Read the model definition and answer for the solid it produces. Units are mm, in the model's axes. A direction names the side the tool comes from. Give positions to 0.01 mm unless a question says otherwise; leave off trailing zeros. Order: outer loops, then holes, each group sorted by start corner. A loop starts at its lowest first (then second) coordinate and runs counter-clockwise, first axis right, second up. Notation, with made-up numbers: (64.5, 42.5) - (70.5, 42.5) arc R22 ccw to (70.5, 69.5) - close; hole circle Ø7 at (-3, 84.5). An arc over 180 degrees is marked (long way). Return JSON: item names as keys, results as strings.
```python
from build123d import *

# Parameters (mm, degrees)
SKETCH_1_R           = 10
EXTRUDE_1_DEPTH      = 250
SKETCH_3_W           = 1.3
SKETCH_3_H           = 0.5
SKETCH_4_OUTSIDE_W   = 122.16
SKETCH_4_OUTSIDE_H   = 122.16
SKETCH_4_OUTSIDE_W_2 = 15
SKETCH_4_OUTSIDE_H_2 = 51.001115416
CUT_EXTRUDE_1_DEPTH  = 10


with BuildPart() as part:
    # 草图1 → 凸台-拉伸1 (new, symmetric)
    with BuildSketch(Plane.XY):
        Circle(SKETCH_1_R)
    extrude(amount=EXTRUDE_1_DEPTH, both=True)

    # 草图3 → 切除-旋转1 (revolve, cut)
    with BuildSketch(Plane(origin=(100, 0, 250), x_dir=(0, 0, -1), z_dir=(0, 1, 0))):
        with Locations((24.45, 90.25)):
            Rectangle(SKETCH_3_W, SKETCH_3_H)
    cut_revolve_1 = revolve(axis=Axis((0, 0, 250), (0, 0, -1)), mode=Mode.SUBTRACT)

    # 草图4 outside → 切除-拉伸1 (cut)
    with BuildSketch(Plane(origin=(0, 0, -250), x_dir=(-1, 0, 0), z_dir=(0, 0, -1))):
        Rectangle(SKETCH_4_OUTSIDE_W, SKETCH_4_OUTSIDE_H)
        Rectangle(SKETCH_4_OUTSIDE_W_2, SKETCH_4_OUTSIDE_H_2, mode=Mode.SUBTRACT)
    cut_extrude_1 = extrude(amount=-CUT_EXTRUDE_1_DEPTH, mode=Mode.SUBTRACT)

    # 镜向1: 切除-旋转1, 切除-拉伸1 across plane
    add(cut_revolve_1.mirror(Plane.XY), mode=Mode.SUBTRACT)
    add(cut_extrude_1.mirror(Plane.XY), mode=Mode.SUBTRACT)


solid = part.part
```
Q1. Consider L1, parallel to X at y = 0.75, z = -29.5; L2, parallel to Y at x = 6.5, z = 188; L3, parallel to Y at x = -7.5, z = 171.5. Determine where each line is inside the solid, lowest interval first.
Values:
{"L1": "x = -9.97 to 9.97", "L2": "y = -7.6 to 7.6", "L3": "y = -6.61 to 6.61"}
Q2. Determine the mould class of faces 6 (the flat face through (9, 4, -226.2)), 7 (the cylindrical face through (-1.302, 9.915, -235.289)), 8 (the flat face through (0, 0, -250)) for opening direction Z: released by +Z, released by -Z, zero draft, split by the parting line, or undercut.
Values:
{"face 6": "undercut", "face 7": "zero draft", "face 8": "released by -Z"}
Q3. A cutting plane is placed at A-A (z = -213). Write down the section's boundary in (x, y).
Values:
{"outline": "circle Ø20 at (0, 0)"}
Q4. Given pin 1 (5 mm diameter, centred on y = 0.5, z = -245.5, fed in from -X); pin 2 (1.2 mm diameter, centred on x = -8.5, y = 0, fed in from -Z); pin 3 (1 mm diameter, centred on x = -7.5, z = -110.5, fed in from -Y), each flat-ended and moving along its own axis, determine where each tip first touches the part or whether it passes through.
Values:
{"pin 1": "stops at x = -7.5", "pin 2": "stops at z = -240", "pin 3": "stops at y = -7.14"}
Q5. For faces 1 (the flat face through (-7.5, 0, 245)), 2 (the flat face through (7.5, 0, -245)), 3 (the flat face through (-7.5, 0, -245)), 4 (the flat face through (7.5, 0, 245)), 5 (the cylindrical face through (4.38, 8.43, -225.54)), determine the directions among +Z, -Z, +X, -X, +Y, -Y from which every point of the face is accessible in a straight line to the end or side of a thin tool.
Values:
{"face 1": "+Z, -X, +Y, -Y", "face 2": "-Z, +X, +Y, -Y", "face 3": "-Z, -X, +Y, -Y", "face 4": "+Z, +X, +Y, -Y", "face 5": "none"}
